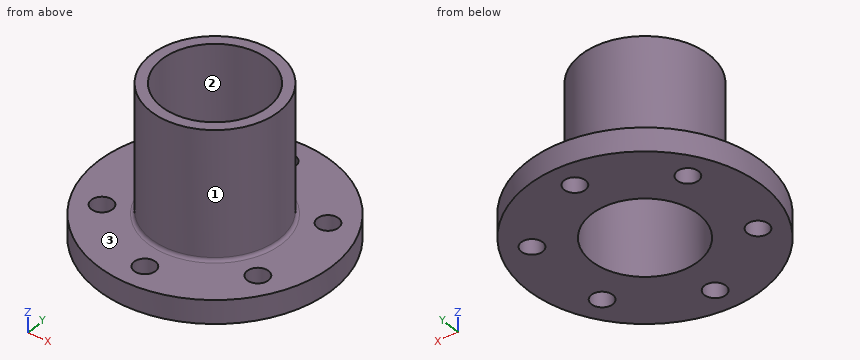
```python
from build123d import *

# Parameters (mm, degrees)
SKETCH2_R           = 110
BOSS_EXTRUDE1_DEPTH = 22
SKETCH3_R           = 60
BOSS_EXTRUDE2_DEPTH = 120
SKETCH4_R           = 50
CUT_EXTRUDE1_DEPTH  = 143
SKETCH5_R           = 10
CUT_EXTRUDE2_DEPTH  = 23
FILLET1_R           = 3


with BuildPart() as part:
    # Sketch2 → Boss-Extrude1 (new body)
    with BuildSketch(Plane.XY):
        Circle(SKETCH2_R)
    extrude(amount=BOSS_EXTRUDE1_DEPTH)

    # Sketch3 → Boss-Extrude2 (add)
    with BuildSketch(Plane.XY.offset(22)):
        Circle(SKETCH3_R)
    extrude(amount=BOSS_EXTRUDE2_DEPTH)

    # Sketch4 → Cut-Extrude1 (cut, through all)
    with BuildSketch(Plane.XY.offset(142)):
        Circle(SKETCH4_R)
    extrude(amount=-CUT_EXTRUDE1_DEPTH, mode=Mode.SUBTRACT)

    # Sketch5 → Cut-Extrude2 (cut, through all)
    with BuildSketch(Plane.XY.offset(22)):
        with Locations((0, 85)):
            Circle(SKETCH5_R)
        with Locations((73.612159322, 42.5)):
            Circle(SKETCH5_R)
        with Locations((73.612159322, -42.5)):
            Circle(SKETCH5_R)
        with Locations((0, -85)):
            Circle(SKETCH5_R)
        with Locations((-73.612159322, -42.5)):
            Circle(SKETCH5_R)
        with Locations((-73.612159322, 42.5)):
            Circle(SKETCH5_R)
    extrude(amount=-CUT_EXTRUDE2_DEPTH, mode=Mode.SUBTRACT)

    # Fillet1
    fillet1_edges = [part.edges().sort_by_distance(p)[0] for p in [
        (-60, 0, 22),
    ]]
    fillet(fillet1_edges, radius=FILLET1_R)


solid = part.part
```
Read the model definition and answer for the solid it produces. Units are mm, in the model's axes. Face numbers are marked on the shaded views. Coordinates: 2 decimals unless noted, no trailing zeros. Order: outer loops, then holes, each group sorted by start corner. A loop starts at its lowest first (then second) coordinate and runs counter-clockwise, first axis right, second up. Notation, with made-up numbers: (17, -19) - (29, -19) arc R17 cw to (29, -5) - close; hole circle Ø4 at (70.25, -5). An arc over 180 degrees is marked (long way). Answer as a JSON object with one key per item and string values. Group by question number.
Item 1: Section C-C (z = 84) is taken. Give the vertices of the cut face in (x, y).
Item 2: The mould has two halves that part along Y. Classify the marked faces 1, 2 and 3: +Y half, -Y half, draft (parallel to the pull), parting line (faces both ways), or undercut.
Item 3: Section B-B (y = 0) is taken. Give the vertices of the cut face in (x, z), plus the area to 3 significant figures.
Item 4: Flat-ended cylindrical pins translate along their axes: P1, Ø6, axis at y = 43.5, z = 18.5, coming from the -X side; P2, Ø10, axis at x = -5, z = 67, coming from the -Y side; P3, Ø8, axis at y = -14.5, z = 67.5, coming from the +X side. Find the tip coordinate at first contact, or state that the pin passes through.
Item 5: Section A-A (x = 0) is taken. Give the vertices of the cut face in (y, z).
Item 6: Section D-D (y = 42.5) is taken. State how many separate pieces and enclosed holes the cut face has, plus the area to 3 significant figures.
Item 7: Consider probe 1 along X at (y, z) = (-42, 16); probe 2 along Y at (x, z) = (1.5, 73.5); probe 3 along Z at (x, y) = (45.5, -45.5). Determine where each line is inside the solid, lowest interval first. Write a range as from..to.
Results are:
{
 "1": {"outline": "circle Ø120 at (0, 0); hole circle Ø100 at (0, 0)"},
 "2": {"face 1": "parting line", "face 2": "undercut", "face 3": "draft"},
 "3": {"outline": "(-110, 0) - (-50, 0) - (-50, 142) - (-60, 142) - (-60, 25) arc R3 cw to (-63, 22) - (-110, 22) - close; (50, 0) - (110, 0) - (110, 22) - (63, 22) arc R3 cw to (60, 25) - (60, 142) - (50, 142) - close", "area": "5,040 mm^2"},
 "4": {"P1": "stops at x = -102.27", "P2": "stops at y = -60", "P3": "stops at x = 59.07"},
 "5": {"outline": "(-110, 0) - (-95, 0) - (-95, 22) - (-110, 22) - close; (-75, 0) - (-50, 0) - (-50, 142) - (-60, 142) - (-60, 25) arc R3 cw to (-63, 22) - (-75, 22) - close; (50, 0) - (75, 0) - (75, 22) - (63, 22) arc R3 cw to (60, 25) - (60, 142) - (50, 142) - close; (95, 0) - (110, 0) - (110, 22) - (95, 22) - close"},
 "6": {"separate pieces": "4", "enclosed holes": "0", "area": "6,270 mm^2"},
 "7": {"probe 1": "x = -101.67..-83.6, -63.62..-27.13, 27.13..63.62, 83.6..101.67", "probe 2": "y = -59.98..-49.98, 49.98..59.98", "probe 3": "z = 0..22"}
}
